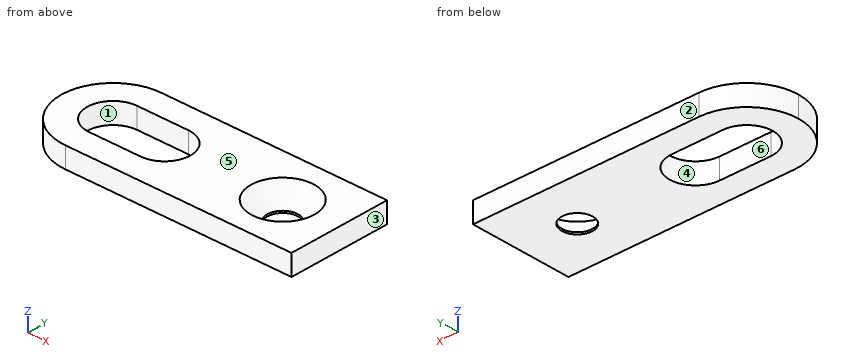
from build123d import *

# Parameters (mm, degrees)
F1_DEPTH       = 2.54
F3_DEPTH       = 2.541
F5_D           = 3.7973
F5_CSINK_D     = 7.7978
F5_CSINK_ANGLE = 82


with BuildPart() as f1:
    # F0 (on Top) → F1 (new body)
    with BuildSketch(Plane.XY):
        with BuildLine():
            ThreePointArc((0, 6.35), (1.8598719395, 1.8598719395), (6.35, 0))
            Line((6.35, 0), (34.29, 0))
            Line((34.29, 0), (34.29, 12.7))
            Line((34.29, 12.7), (6.35, 12.7))
            ThreePointArc((6.35, 12.7), (1.8598719395, 10.8401280605), (0, 6.35))
        make_face()
    extrude(amount=F1_DEPTH)

    # F2 (on face) → F3 (cut, through all)
    with BuildSketch(Plane.XY.offset(2.54)):
        with BuildLine():
            Line((12.7, 9.525), (6.35, 9.525))
            ThreePointArc((6.35, 9.525), (3.175, 6.35), (6.35, 3.175))
            Line((6.35, 3.175), (12.7, 3.175))
            ThreePointArc((12.7, 3.175), (15.875, 6.35), (12.7, 9.525))
        make_face()
    extrude(amount=-F3_DEPTH, mode=Mode.SUBTRACT)

    # F5 (through all)
    with Locations(Plane.XY.offset(2.54)):
        with Locations((27.305, 6.35)):
            CounterSinkHole(F5_D / 2, F5_CSINK_D / 2, counter_sink_angle=F5_CSINK_ANGLE)


solid = f1.part
For this review, take the finished solid that the model builds, in its own axes (mm). Face numbers are marked on the shaded views. A direction names the side the tool comes from. Give positions to 0.01 mm unless a question says otherwise; leave off trailing zeros. Loops run counter-clockwise (first coordinate to the right, second up) from the corner with the lowest first, then second, coordinate; pieces in that order, holes last. Notation, with made-up numbers: M 45.25,-10.5 L 76.25,-10.5 A24 cw 76.25,10.5 Z; hole C 5.25,61 d6. An arc over 180 degrees is marked long. Answer as a JSON object with one key per item and string values. Group by question number.
Q1. For probe 1 along X at (y, z) = (6.35, 0.2) (3 decimals); probe 2 along X at (y, z) = (8.25, 1.35); probe 3 along Y at (x, z) = (10, 2) (3 decimals), list the stretches that pass through material, from the lowest coordinate up. Write a range as [from, to].
Q2. Tool access review of the marked faces 5 and 6: name each direction out of +Z, -Z, +X, -X, +Y, -Y from which nothing blocks a thin tool from reaching the whole face with its end or side.
Q3. Add section A-A on x = 10.5. Give the boundary of the cut face in (y, z) (3 decimals), and give its area (3 significant figures).
Q4. Add section C-C on y = 6.75. Give the number of separate pieces and of enclosed holes in the cut face, and give its area (3 significant figures).
Q5. Add section B-B on z = 1.05. Give the boundary of the cut face in (x, y) (3 decimals).
Q6. Mouldability with a two-part tool opening along X and no side actions: class the marked faces 1, 2, 3 and 4 as +X half, -X half, draft (parallel to the pull), parting line (faces both ways), or undercut.
Checked values:
{
 "1": {"probe 1": "[0, 3.175], [15.875, 25.406], [29.204, 34.29]", "probe 2": "[0.29, 3.81], [15.24, 25.16], [29.45, 34.29]", "probe 3": "[0, 3.175], [9.525, 12.7]"},
 "2": {"face 5": "+Z, +X, -X, +Y, -Y", "face 6": "+Z, -Z"},
 "3": {"outline": "M 0,0 L 3.175,0 L 3.175,2.54 L 0,2.54 Z; M 9.525,0 L 12.7,0 L 12.7,2.54 L 9.525,2.54 Z", "area": "16.1 mm²"},
 "4": {"separate pieces": "3", "enclosed holes": "0", "area": "40.8 mm²"},
 "5": {"outline": "M 6.35,0 L 34.29,0 L 34.29,12.7 L 6.35,12.7 A6.35 ccw Z; hole M 6.35,3.175 L 12.7,3.175 A3.175 ccw 12.7,9.525 L 6.35,9.525 A3.175 ccw Z; hole C 27.305,6.35 d5.207"},
 "6": {"face 1": "undercut", "face 2": "draft", "face 3": "+X half", "face 4": "undercut"}
}
